from build123d import *

# Parameters (mm, degrees)
SKETCH_1_R          = 1.55
SKETCH_1_W          = 9.95
SKETCH_1_H          = 2.5
EXTRUDE_1_DEPTH     = 1
SKETCH_2_R          = 0.75
CUT_EXTRUDE_1_DEPTH = 3
CUT_EXTRUDE_2_DEPTH = 3
SKETCH_4_R          = 0.75
CUT_EXTRUDE_3_DEPTH = 3


with BuildPart() as part:
    # 草图1 → 凸台-拉伸1 (new body, symmetric)
    with BuildSketch(Plane.XY):
        Polygon((-30.025, 1.25), (-30.025, -2.5), (-34.051193345, -8.25), (-45.948806655, -8.25), (-49.975, -2.5), (-49.975, 2.5), (-45.948806655, 8.25), (45.948806655, 8.25), (49.975, 2.5), (49.975, -2.5), (45.948806655, -8.25), (34.051193345, -8.25), (30.025, -2.5), (30.025, 1.25), align=None)
        with Locations((-40, 4.75)):
            Circle(SKETCH_1_R, mode=Mode.SUBTRACT)
        with Locations((-40, -4.75)):
            Circle(SKETCH_1_R, mode=Mode.SUBTRACT)
        with Locations((40, -4.75)):
            Circle(SKETCH_1_R, mode=Mode.SUBTRACT)
        with Locations((40, 4.75)):
            Circle(SKETCH_1_R, mode=Mode.SUBTRACT)
        with Locations((-40, 0)):
            Rectangle(SKETCH_1_W, SKETCH_1_H, mode=Mode.SUBTRACT)
        with Locations((40, 0)):
            Rectangle(SKETCH_1_W, SKETCH_1_H, mode=Mode.SUBTRACT)
    extrude(amount=EXTRUDE_1_DEPTH, both=True)

    # 草图2 → 切除-拉伸1 (cut, through all)
    with BuildSketch(Plane.XY.offset(1)):
        with Locations((-35.775, 1.25)):
            Circle(SKETCH_2_R)
        with Locations((-35.775, -1.25)):
            Circle(SKETCH_2_R)
        with Locations((-44.225, 1.25)):
            Circle(SKETCH_2_R)
        with Locations((-44.225, -1.25)):
            Circle(SKETCH_2_R)
        with Locations((-29.275, 1.25)):
            Circle(SKETCH_2_R)
        with Locations((29.275, 1.25)):
            Circle(SKETCH_2_R)
        with Locations((44.225, -1.25)):
            Circle(SKETCH_2_R)
        with Locations((44.225, 1.25)):
            Circle(SKETCH_2_R)
        with Locations((35.775, -1.25)):
            Circle(SKETCH_2_R)
        with Locations((35.775, 1.25)):
            Circle(SKETCH_2_R)
    extrude(amount=-CUT_EXTRUDE_1_DEPTH, mode=Mode.SUBTRACT)

    # 草图3 → 切除-拉伸2 (cut, through all)
    with BuildSketch(Plane.XY.offset(1)):
        Polygon((-30, 8.25), (-27.616492815, 6.25), (27.616492815, 6.25), (30, 8.25), align=None)
    extrude(amount=-CUT_EXTRUDE_2_DEPTH, mode=Mode.SUBTRACT)

    # 草图4 → 切除-拉伸3 (cut, through all)
    with BuildSketch(Plane.XY.offset(1)):
        with Locations((-27.134402108, 6.824533332)):
            Circle(SKETCH_4_R)
        with Locations((27.134402108, 6.824533332)):
            Circle(SKETCH_4_R)
    extrude(amount=-CUT_EXTRUDE_3_DEPTH, mode=Mode.SUBTRACT)


solid = part.part
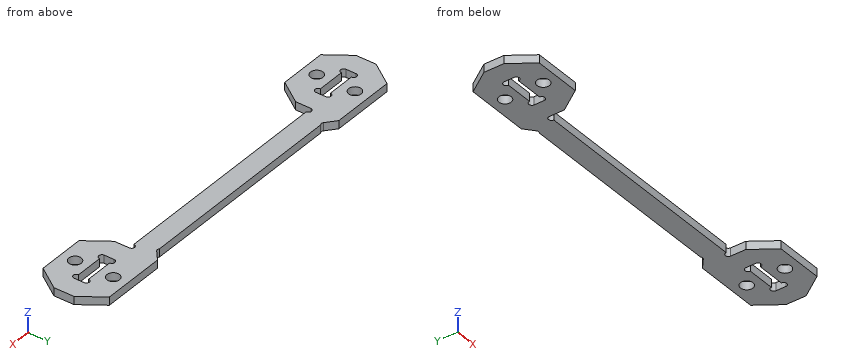
Check sheet for the modelled part. Datum: model origin and axes. Units: mm. Give positions to 0.01 mm unless a question says otherwise; leave off trailing zeros. Loops run counter-clockwise (first coordinate to the right, second up) from the corner with the lowest first, then second, coordinate; pieces in that order, holes last. Notation, with made-up numbers: M 73,56 L 87,56 A26 cw 87,85 Z; hole C 45.25,54 d6. An arc over 180 degrees is marked long. Return JSON: item names as keys, results as strings. Group by question number.
1. Cross-section at C-C on z = -0.1. State how many separate pieces and enclosed holes the cut face has, plus the area to 3 significant figures.
2. Cross-section at A-A on x = 40. Record the boundary of the cut face in (y, z).
3. Cross-section at D-D on x = 16.5. Record the boundary of the cut face in (y, z), plus the area to 3 significant figures.
4. Thickness scan on L1, parallel to Y at x = -40, z = 0.05; L2, parallel to X at y = -1.5, z = 0.9 (3 decimals); L3, parallel to X at y = -5.75, z = 0.45. Record the ranges inside material, lowest first.
5. Go/stop test with a flat-tipped pin: pin 1 (3 mm diameter, centred on x = -40, y = -4.75, fed in from -Z). Record where the tip stops, or that it passes through.
6. Cross-section at B-B on y = -4.75. Record the boundary of the cut face in (x, z), plus the area to 3 significant figures.
Return value:
{
 "1": {"separate pieces": "1", "enclosed holes": "6", "area": "805 mm^2"},
 "2": {"outline": "M -8.25,-1 L -6.3,-1 L -6.3,1 L -8.25,1 Z; M -3.2,-1 L -1.25,-1 L -1.25,1 L -3.2,1 Z; M 1.25,-1 L 3.2,-1 L 3.2,1 L 1.25,1 Z; M 6.3,-1 L 8.25,-1 L 8.25,1 L 6.3,1 Z"},
 "3": {"outline": "M 1.25,-1 L 6.25,-1 L 6.25,1 L 1.25,1 Z", "area": "10.0 mm^2"},
 "4": {"L1": "-8.25 to -6.3, -3.2 to -1.25, 1.25 to 3.2, 6.3 to 8.25", "L2": "-49.975 to -44.932, -43.518 to -36.482, -35.068 to -30.025, 30.025 to 35.068, 36.482 to 43.518, 44.932 to 49.975", "L3": "-47.7 to -41.18, -38.82 to -32.3, 32.3 to 38.82, 41.18 to 47.7"},
 "5": {"pin 1": "through"},
 "6": {"outline": "M -48.4,-1 L -41.55,-1 L -41.55,1 L -48.4,1 Z; M -38.45,-1 L -31.6,-1 L -31.6,1 L -38.45,1 Z; M 31.6,-1 L 38.45,-1 L 38.45,1 L 31.6,1 Z; M 41.55,-1 L 48.4,-1 L 48.4,1 L 41.55,1 Z", "area": "54.8 mm^2"}
}
